For this review, take the finished solid that the model builds, in its own axes (mm). A direction names the side the tool comes from. Give positions to 0.01 mm unless a question says otherwise; leave off trailing zeros. Write each loop counter-clockwise with the first axis right and the second up, starting at its lowest first coordinate (ties: lowest second). Pieces come first, ordered by that corner, then holes.
from build123d import *

# Parameters (mm, degrees)
F0_W     = 22.86
F0_H     = 22.86
F0_W_2   = 12.954
F0_H_2   = 12.954
F1_DEPTH = 25.4
F2_DEPTH = 22.86
F3_W     = 12.954
F3_H     = 12.954
F4_DEPTH = 5.08
F5_W     = 12.9547669124
F5_H     = 12.7
F6_DEPTH = 25.4


with BuildPart() as f1:
    # F0 (on Right) → F1 (new body)
    with BuildSketch(Plane.YZ):
        Rectangle(F0_W, F0_H)
        Rectangle(F0_W_2, F0_H_2, mode=Mode.SUBTRACT)
    extrude(amount=F1_DEPTH)

    # F2 (add): a face of the model
    f2_faces = [f1.faces().sort_by_distance(p)[0] for p in [
        (12.7, 11.43, 0),
    ]]
    extrude(f2_faces, amount=F2_DEPTH)

    # F3 (on face) → F4 (join)
    with BuildSketch(Plane.YZ.offset(25.4)):
        Rectangle(F3_W, F3_H)
    extrude(amount=-F4_DEPTH)

    # F5 (on face) → F6 (cut)
    with BuildSketch(Plane(origin=(0, 34.29, 0), x_dir=(-1, 0, 0), z_dir=(0, 1, 0))):
        with Locations((-11.5566165438, 0)):
            Rectangle(F5_W, F5_H)
    extrude(amount=-F6_DEPTH, mode=Mode.SUBTRACT)


solid = f1.part
(1) Clearance check with flat-ended pins moving along their axes: pin 1 Ø4 at (y, z) = (-2.5, 0) entering from -X; pin 2 Ø6.5 at (x, z) = (12, 0.5) entering from +Y. State where each tip first meets the part, or that it passes through.
(2) Tool access review of faces 4 (the flat face through (13, 11, -11.43)), 5 (the flat face through (10, 6.477, 0)), 6 (the flat face through (12, 8.89, 0)): name each direction out of +Z, -Z, +X, -X, +Y, -Y from which nothing blocks a thin tool from reaching the whole face with its end or side.
(3) We need section A-A (y = 18). Write out the cut boundary in (x, z).
(4) For L1, parallel to Y at x = 1.5, z = -6; L2, parallel to Z at x = 4.25, y = -1.5; L3, parallel to Y at x = 13, z = 0.75, list the stretches that pass through material, from the lowest coordinate up.
(5) We need section B-B (x = 19). Write out the cut boundary in (y, z), and give its area (3 significant figures).
(6) We need section D-D (y = 4). Write out the cut boundary in (x, z).
(7) We need section C-C (z = 5.25). Write out the cut boundary in (x, y).
(8) The part is to be moulded in two halves that separate along Z. For faces 1 (the flat face through (18.2, 34.29, -0.2)), 2 (the flat face through (10, -6.477, 0)), 3 (the flat face through (13, 11, 11.43)), say which applies: +Z half, -Z half, draft (parallel to the pull), parting line (faces both ways), or undercut.
The answers:
1. pin 1: stops at x = 20.32
1. pin 2: stops at y = 8.89
2. face 4: -Z, +X, -X, +Y, -Y
2. face 5: -X
2. face 6: +Y
3. outline: (0, -11.43) - (25.4, -11.43) - (25.4, 11.43) - (0, 11.43) - close; hole (5.08, -6.35) - (18.03, -6.35) - (18.03, 6.35) - (5.08, 6.35) - close
4. L1: y = -11.43 to -6.48, 6.48 to 34.29
4. L2: z = -11.43 to -6.48, 6.48 to 11.43
4. L3: y = -11.43 to -6.48, 6.48 to 8.89
5. outline: (-11.43, -11.43) - (34.29, -11.43) - (34.29, 11.43) - (-11.43, 11.43) - close; hole (-6.48, -6.48) - (6.48, -6.48) - (6.48, 6.48) - (-6.48, 6.48) - close
5. area: 877 mm2
6. outline: (0, -11.43) - (25.4, -11.43) - (25.4, 11.43) - (0, 11.43) - (0, 6.48) - (20.32, 6.48) - (20.32, -6.48) - (0, -6.48) - close
7. outline: (0, -11.43) - (25.4, -11.43) - (25.4, 34.29) - (18.03, 34.29) - (18.03, 8.89) - (5.08, 8.89) - (5.08, 34.29) - (0, 34.29) - (0, 6.48) - (20.32, 6.48) - (20.32, -6.48) - (0, -6.48) - close
8. face 1: draft
8. face 2: undercut
8. face 3: +Z half
